```python
from build123d import *

# Parameters (mm, degrees)
SKETCH_1_W               = 45
SKETCH_1_H               = 5
EXTRUDE_1_DEPTH          = 242.8
CUT_EXTRUDE_2_DEPTH      = 244.891553769
CUT_EXTRUDE_2_DEPTH_BACK = 244.891553769
SKETCH_3_R               = 3.5
CUT_EXTRUDE_3_DEPTH      = 247.947545037
CUT_EXTRUDE_3_DEPTH_BACK = 247.947545037


with BuildPart() as part:
    # Эскиз1 → Бобышка-Вытянуть1 (new body)
    with BuildSketch(Plane.XY):
        Rectangle(SKETCH_1_W, SKETCH_1_H)
    extrude(amount=EXTRUDE_1_DEPTH)

    # Эскиз3 → Вырез-Вытянуть2 (cut, two sides: drawn at the far end of the back side and taken through both)
    with BuildSketch(Plane(origin=(0, 2.5, 0), x_dir=(1, 0, 0), z_dir=(0, 1, 0)).offset(-CUT_EXTRUDE_2_DEPTH_BACK)):
        with Locations(Location((0, -42, 0), (0, 0, 270))):
            Circle(SKETCH_3_R)
        with Locations(Location((0, -182, 0), (0, 0, 270))):
            Circle(SKETCH_3_R)
        with Locations((0, -322)):
            Circle(SKETCH_3_R)
        with Locations((0, -462)):
            Circle(SKETCH_3_R)
        with Locations((0, -602)):
            Circle(SKETCH_3_R)
        with Locations((0, -742)):
            Circle(SKETCH_3_R)
        with Locations((0, -882)):
            Circle(SKETCH_3_R)
        with Locations((0, -1022)):
            Circle(SKETCH_3_R)
        with Locations((0, -1162)):
            Circle(SKETCH_3_R)
        with Locations((0, -1302)):
            Circle(SKETCH_3_R)
    extrude(amount=CUT_EXTRUDE_2_DEPTH + CUT_EXTRUDE_2_DEPTH_BACK, mode=Mode.SUBTRACT)

    # Эскиз4 → Вырез-Вытянуть3 (cut, two sides: drawn at the far end of the back side and taken through both)
    with BuildSketch(Plane.ZY.offset(22.5).offset(-CUT_EXTRUDE_3_DEPTH_BACK)):
        Polygon((242.8, -2.5), (224.139745962, 2.5), (242.8, 2.5), align=None)
    extrude(amount=CUT_EXTRUDE_3_DEPTH + CUT_EXTRUDE_3_DEPTH_BACK, mode=Mode.SUBTRACT)


solid = part.part
```
Geometry check sheet. Reference: the model listing, model coordinates, mm. Give positions to 0.01 mm unless a question says otherwise; leave off trailing zeros. Loops run counter-clockwise (first coordinate to the right, second up) from the corner with the lowest first, then second, coordinate; pieces in that order, holes last. Notation, with made-up numbers: M -35,11 L 23,11 A28 cw 23,35 Z; hole C 9,32 d10. An arc over 180 degrees is marked long. Answer as CSV lines item,"result".
Item 1: Release check for a two-part mould opening along Z. For faces 1 (the flat face through (0, 0, 0)), 2 (the flat face through (-22.5, 0, 120)), 3 (the cylindrical face through (1.05, -0.03, 185.34)) record: pulls with the +Z half, pulls with the -Z half, needs draft (parallel to the pull), parting line crosses it, or undercut.
Values:
face 1,"pulls with the -Z half"
face 2,"needs draft"
face 3,"undercut"
Item 2: Material ranges on line 1 (X direction, y = 1.15, z = 182); line 2 (X direction, y = -1.25, z = 43.5), recorded low to high.
Values:
line 1,"x = -22.5 to -3.5, 3.5 to 22.5"
line 2,"x = -22.5 to -3.16, 3.16 to 22.5"
Item 3: Cross-section at A-A on x = 0. Record the cut outline in (y, z), and give its area (3 significant figures).
Values:
outline,"M -2.5,0 L 2.5,0 L 2.5,38.5 L -2.5,38.5 Z; M -2.5,45.5 L 2.5,45.5 L 2.5,178.5 L -2.5,178.5 Z; M -2.5,185.5 L 2.5,185.5 L 2.5,224.14 L -2.5,242.8 Z"
area,"1,100 mm²"
Item 4: Cross-section at D-D on x = -15. Record the cut outline in (y, z), and give its area (3 significant figures).
Values:
outline,"M -2.5,0 L 2.5,0 L 2.5,224.14 L -2.5,242.8 Z"
area,"1,170 mm²"
Item 5: Depth check by flat-ended pin: P1, Ø9, axis at x = 0, z = 42, coming from the -Y side. Enter the tip coordinate at first touch or a pass-through.
Values:
P1,"stops at y = -2.5"
Item 6: Cross-section at C-C on y = -1.35. Record the cut outline in (x, z), and give its area (3 significant figures).
Values:
outline,"M -22.5,0 L 22.5,0 L 22.5,238.51 L -22.5,238.51 Z; hole C 0,42 d7; hole C 0,182 d7"
area,"10,700 mm²"
Item 7: Cross-section at B-B on z = 182. Record the cut outline in (x, y), and give its area (3 significant figures).
Values:
outline,"M -22.5,-2.5 L -3.5,-2.5 L -3.5,2.5 L -22.5,2.5 Z; M 3.5,-2.5 L 22.5,-2.5 L 22.5,2.5 L 3.5,2.5 Z"
area,"190 mm²"
